Geometry: final body of the model. Coordinates: model frame, mm. Give positions to 0.01 mm unless a question says otherwise; leave off trailing zeros. Loops run counter-clockwise (first coordinate to the right, second up) from the corner with the lowest first, then second, coordinate; pieces in that order, holes last. Notation, with made-up numbers: M 43,52 L 69,52 A18 ccw 69,85 Z; hole C 54.5,-8.5 d10. An arc over 180 degrees is marked long. Put each result on its own line as item: value.
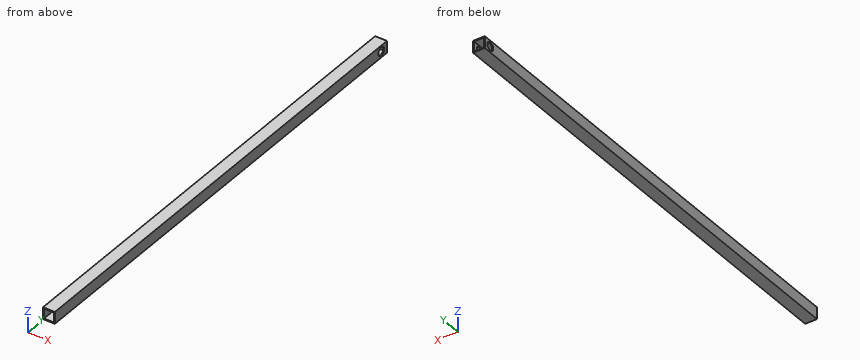
```python
from build123d import *

# Parameters (mm, degrees)
SKETCH1_W           = 38.1
SKETCH1_H           = 38.1
SKETCH1_W_2         = 31.75
SKETCH1_H_2         = 31.75
BOSS_EXTRUDE1_DEPTH = 1524
CUT_EXTRUDE1_DEPTH  = 38.1


with BuildPart() as part:
    # Sketch1 → Boss-Extrude1 (new body)
    with BuildSketch(Plane(origin=(0, 0, 0), x_dir=(1, 0, 0), z_dir=(0, 1, 0))):
        with Locations((19.05, 19.05)):
            Rectangle(SKETCH1_W, SKETCH1_H)
        with Locations((19.05, 19.05)):
            Rectangle(SKETCH1_W_2, SKETCH1_H_2, mode=Mode.SUBTRACT)
    extrude(amount=BOSS_EXTRUDE1_DEPTH)

    # Sketch2 → Cut-Extrude1 (cut)
    with BuildSketch(Plane(origin=(38.1, 0, 0), x_dir=(0, 0, -1), z_dir=(1, 0, 0))):
        Polygon((33.714696837, 1498.6), (26.382348419, 1511.3), (11.717651581, 1511.3), (4.385303163, 1498.6), (11.717651581, 1485.9), (26.382348419, 1485.9), align=None)
    extrude(amount=-CUT_EXTRUDE1_DEPTH, mode=Mode.SUBTRACT)


solid = part.part
```
Item 1: Line query: probe 1 along X at (y, z) = (947.5, -7) (3 decimals); probe 2 along Z at (x, y) = (11, 848.5) (3 decimals); probe 3 along Y at (x, z) = (2, -18). Output: solid intervals per line, ascending. Write a range as [from, to].
Output values:
probe 1: [0, 3.175], [34.925, 38.1]
probe 2: [-38.1, -34.925], [-3.175, 0]
probe 3: [0, 1485.9], [1511.3, 1524]
Item 2: Section B-B on y = 1133.5. Output: boundary loops of the cut face in (x, z) (3 decimals), then the cut area to 3 significant figures.
Output values:
outline: M 0,-38.1 L 38.1,-38.1 L 38.1,0 L 0,0 Z; hole M 3.175,-34.925 L 34.925,-34.925 L 34.925,-3.175 L 3.175,-3.175 Z
area: 444 mm²
Item 3: Section A-A on x = 28.5. Output: boundary loops of the cut face in (y, z) (3 decimals), then the cut area to 3 significant figures.
Output values:
outline: M 0,-38.1 L 1524,-38.1 L 1524,-34.925 L 0,-34.925 Z; M 0,-3.175 L 1524,-3.175 L 1524,0 L 0,0 Z
area: 9,680 mm²
